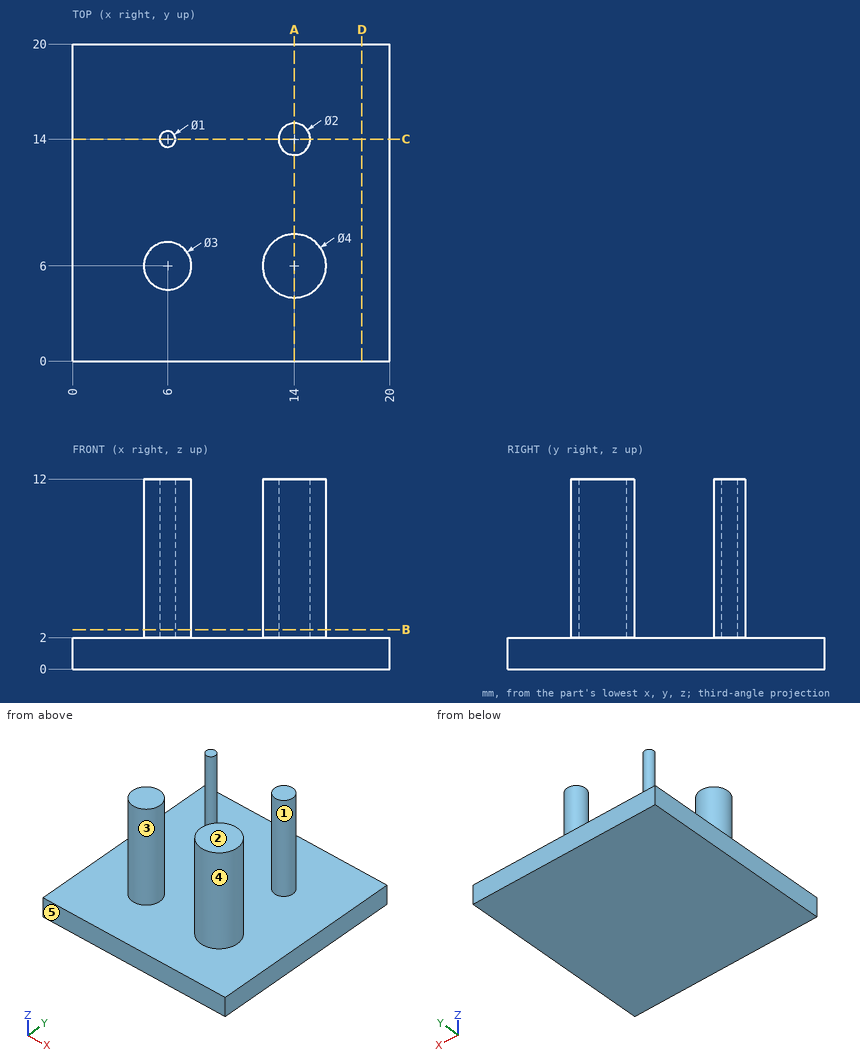
Answer from the drawing. Dimensions are ordinates in mm from the lowest x, y and z of the part. A direction names the side the tool comes from. Coordinates: 2 decimals unless noted, no trailing zeros. Write each loop counter-clockwise with the first axis right and the second up, starting at its lowest first coordinate (ties: lowest second). Pieces come first, ordered by that corner, then holes. Notation, with made-up numbers: (85.25, 30.5) -> (113.25, 30.5) arc R15 cw to (113.25, 42.5) -> close; hole circle Ø6 at (39, -7). An arc over 180 degrees is marked (long way). One line per question, with ' | ' between items.
1. Which of the six approach directions +Z, -Z, +X, -X, +Y, -Y give full straight-line access (tool end or side, diameter ignored) to the marked faces 1 and 2?
Verdict:
face 1: +Z | face 2: +Z, +X, -X, +Y, -Y
2. Straight lines are drawn through the part: line 1 (Z direction, x = 18.75, y = 7); line 2 (X direction, y = 6.75, z = 9); line 3 (Y direction, x = 5.25, z = 7.75). For each, find the intervals that lie inside material, in ascending order.
Verdict:
line 1: z = 0 to 2 | line 2: x = 4.7 to 7.3, 12.15 to 15.85 | line 3: y = 4.7 to 7.3
3. Section B-B (z = 2.5) is taken. Determine the outline of the cut face in (x, y), and give its area (3 significant figures).
Verdict:
outline: circle Ø3 at (6, 6); circle Ø1 at (6, 14); circle Ø4 at (14, 6); circle Ø2 at (14, 14) | area: 23.6 mm^2
4. Section D-D (x = 18.25) is taken. Determine the outline of the cut face in (y, z), and give its area (3 significant figures).
Verdict:
outline: (0, 0) -> (20, 0) -> (20, 2) -> (0, 2) -> close | area: 40.0 mm^2
5. Section C-C (y = 14) is taken. Determine the outline of the cut face in (x, z), and give its area (3 significant figures).
Verdict:
outline: (0, 0) -> (20, 0) -> (20, 2) -> (15, 2) -> (15, 12) -> (13, 12) -> (13, 2) -> (6.5, 2) -> (6.5, 12) -> (5.5, 12) -> (5.5, 2) -> (0, 2) -> close | area: 70.0 mm^2
6. Given pin 1 Ø6 at (y, z) = (5.5, 3.5) entering from +X; pin 2 Ø6 at (y, z) = (15.5, 6) entering from +X; pin 3 Ø1 at (x, z) = (13, 8) entering from -Y, each flat-ended and moving along its own axis, determine where each tip first touches the part or whether it passes through.
Verdict:
pin 1: stops at x = 20 | pin 2: stops at x = 15 | pin 3: stops at y = 4.06
7. For a pull along X with two mould halves and no side action, classify the marked faces 3, 4 and 5 as released by +X, released by -X, zero draft, split by the parting line, or undercut.
Verdict:
face 3: undercut | face 4: undercut | face 5: zero draft
8. Section A-A (x = 14) is taken. Determine the outline of the cut face in (y, z).
Verdict:
outline: (0, 0) -> (20, 0) -> (20, 2) -> (15, 2) -> (15, 12) -> (13, 12) -> (13, 2) -> (8, 2) -> (8, 12) -> (4, 12) -> (4, 2) -> (0, 2) -> close
